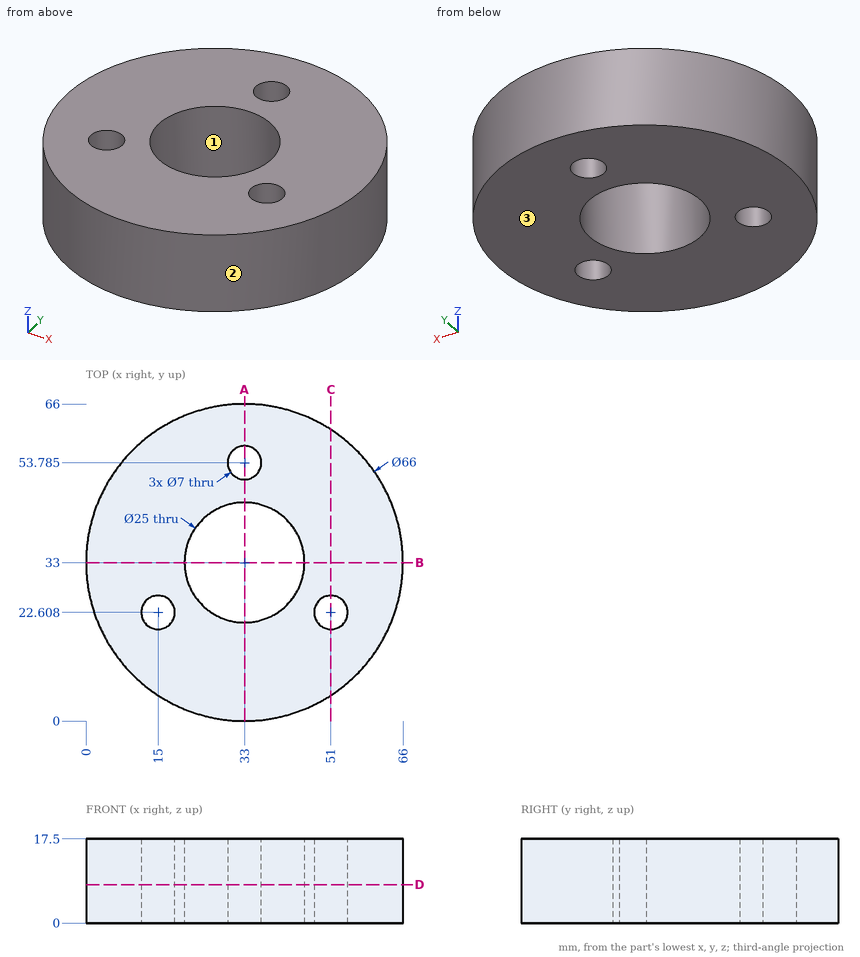
Can you work these out from the drawing? Everything is in mm from the part's minimum corner. Give positions to 0.01 mm unless a question says otherwise; leave off trailing zeros. Order: outer loops, then holes, each group sorted by start corner. A loop starts at its lowest first (then second) coordinate and runs counter-clockwise, first axis right, second up. Notation, with made-up numbers: M 73,20.25 L 123,20.25 A21 ccw 123,32.25 Z; hole C -35,1.25 d6. An arc over 180 degrees is marked long. Use a Markdown table: item, result. Add a question column.
Item 1: Suppose I cut it at D-D (z = 8). List the corners of the cut face in (x, y) for me (1 decimal).
Item 2: Suppose I cut it at A-A (x = 33). List the corners of the cut face in (y, z) for me (1 decimal), then the cut area to 3 significant figures.
Item 3: Suppose I cut it at B-B (y = 33). List the corners of the cut face in (x, z) for me.
Item 4: We'd pull the mould along X, two halves only. Please class the marked faces 1, 2 and 3: +X half, -X half, draft (parallel to the pull), parting line (faces both ways), or undercut.
Item 5: Suppose I cut it at C-C (x = 51). List the corners of the cut face in (y, z) for me.
Item 6: If I drill on L1, parallel to Y at x = 33, z = 6 (1 decimal); L2, parallel to X at y = 22.5, z = 3 (1 decimal); L3, parallel to Y at x = 51, z = 8.75, over which ranges is the centre line in solid material (lowest first)? Write a range as [from, to].
Item 7: Will these pins go through, and if not, where does the flat tip stop? pin 1 (11 mm diameter, centred on x = 33, y = 53.78, fed in from -Z); pin 2 (1 mm diameter, centred on x = 57, z = 15, fed in from +Y); pin 3 (4 mm diameter, centred on x = 51, y = 22.61, fed in from -Z); pin 4 (2 mm diameter, centred on y = 22, z = 8, fed in from -X).
Answer sheet:
| question | item | result |
|---|---|---|
| 1 | outline | C 33,33 d66; hole C 15,22.6 d7; hole C 33,33 d25; hole C 33,53.8 d7; hole C 51,22.6 d7 |
| 2 | outline | M 0,0 L 20.5,0 L 20.5,17.5 L 0,17.5 Z; M 45.5,0 L 50.3,0 L 50.3,17.5 L 45.5,17.5 Z; M 57.3,0 L 66,0 L 66,17.5 L 57.3,17.5 Z |
| 2 | area | 595 mm² |
| 3 | outline | M 0,0 L 20.5,0 L 20.5,17.5 L 0,17.5 Z; M 45.5,0 L 66,0 L 66,17.5 L 45.5,17.5 Z |
| 4 | face 1 | undercut |
| 4 | face 2 | parting line |
| 4 | face 3 | draft |
| 5 | outline | M 5.34,0 L 19.11,0 L 19.11,17.5 L 5.34,17.5 Z; M 26.11,0 L 60.66,0 L 60.66,17.5 L 26.11,17.5 Z |
| 6 | L1 | y = [0, 20.5], [45.5, 50.3], [57.3, 66] |
| 6 | L2 | x = [1.7, 11.5], [18.5, 26.2], [39.8, 47.5], [54.5, 64.3] |
| 6 | L3 | y = [5.34, 19.11], [26.11, 60.66] |
| 7 | pin 1 | stops at z = 0 |
| 7 | pin 2 | stops at y = 56.17 |
| 7 | pin 3 | passes through |
| 7 | pin 4 | stops at x = 1.55 |
